Could you check a few things on this model? Use its own coordinates, in mm. Give positions to 0.01 mm unless a question says otherwise; leave off trailing zeros. Write each loop counter-clockwise with the first axis right and the second up, starting at its lowest first coordinate (ties: lowest second). Pieces come first, ordered by that corner, then holes. Notation, with made-up numbers: (87.5, 49) - (137.5, 49) arc R25 cw to (137.5, 86) - close; hole circle Ø7 at (33, -18). An arc over 180 degrees is marked (long way). Write item = value, one per line.
from build123d import *

# Parameters (mm, degrees)
SKETCH1_W           = 68
SKETCH1_H           = 8.5
BOSS_EXTRUDE1_DEPTH = 5
SKETCH2_W           = 60
SKETCH2_H           = 1.5
CUT_EXTRUDE1_DEPTH  = 3
FILLET1_R           = 2


with BuildPart() as part:
    # Sketch1 → Boss-Extrude1 (new body)
    with BuildSketch(Plane.XY):
        with Locations((34, 4.25)):
            Rectangle(SKETCH1_W, SKETCH1_H)
    extrude(amount=BOSS_EXTRUDE1_DEPTH)

    # Sketch2 → Cut-Extrude1 (cut)
    with BuildSketch(Plane.XY.offset(5)):
        with Locations((34, 4.25)):
            Rectangle(SKETCH2_W, SKETCH2_H)
    extrude(amount=-CUT_EXTRUDE1_DEPTH, mode=Mode.SUBTRACT)

    # Fillet1
    fillet1_edges = [part.edges().sort_by_distance(p)[0] for p in [
        (68, 4.25, 0),
        (0, 4.25, 0),
    ]]
    fillet(fillet1_edges, radius=FILLET1_R)


solid = part.part
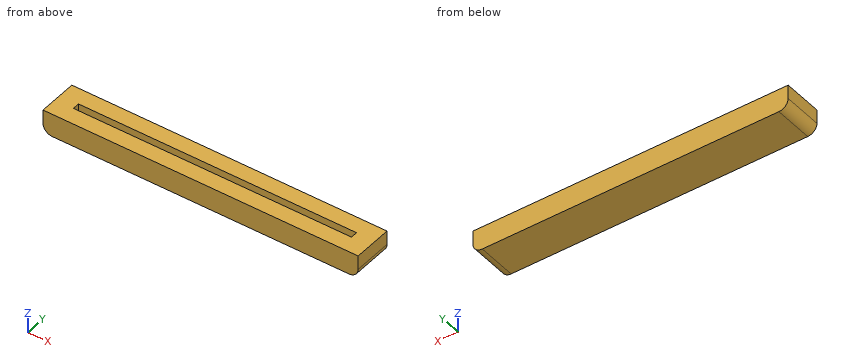
1. If we section it at A-A, the plane z = 4.3: Please give me the cut outline in (x, y).
Filled sheet:
outline = (0, 0) - (68, 0) - (68, 8.5) - (0, 8.5) - close; hole (4, 3.5) - (64, 3.5) - (64, 5) - (4, 5) - close
2. If we section it at B-B, the plane x = 27: Please give me the cut outline in (y, z), and give its area (3 significant figures).
Filled sheet:
outline = (0, 0) - (8.5, 0) - (8.5, 5) - (5, 5) - (5, 2) - (3.5, 2) - (3.5, 5) - (0, 5) - close
area = 38.0 mm2
3. I need wall thicknesses on line 1 (Y direction, x = 29, z = 2.5); line 2 (X direction, y = 4.75, z = 4.6); line 3 (X direction, y = 7, z = 1.8). Which ranges of each line are inside material? Lowest first, please.
Filled sheet:
line_1 = 0 to 3.5, 5 to 8.5
line_2 = 0 to 4, 64 to 68
line_3 = 0.01 to 67.99
